```python
from build123d import *

# Parameters (mm, degrees)
SKETCH_1_R      = 2
EXTRUDE_2_DEPTH = 4


with BuildPart() as part:
    # 草图1 → 凸台-拉伸2 (new body)
    with BuildSketch(Plane(origin=(0, 0, 0), x_dir=(1, 0, 0), z_dir=(0, 1, 0))):
        with BuildLine():
            Line((0, -30), (150, -20))
            ThreePointArc((150, -20), (170, 0), (150, 20))
            Line((150, 20), (0, 30))
            ThreePointArc((0, 30), (-30, 0), (0, -30))
        make_face()
        with Locations(Location((0, -17.25, 0), (0, 0, 270))):
            Circle(SKETCH_1_R, mode=Mode.SUBTRACT)
        with Locations(Location((-14.938938215, -8.625, 0), (0, 0, 270))):
            Circle(SKETCH_1_R, mode=Mode.SUBTRACT)
        with Locations(Location((14.938938215, -8.625, 0), (0, 0, 270))):
            Circle(SKETCH_1_R, mode=Mode.SUBTRACT)
        with Locations(Location((-14.938938215, 8.625, 0), (0, 0, 270))):
            Circle(SKETCH_1_R, mode=Mode.SUBTRACT)
        with Locations(Location((14.938938215, 8.625, 0), (0, 0, 270))):
            Circle(SKETCH_1_R, mode=Mode.SUBTRACT)
        with Locations(Location((0, 17.25, 0), (0, 0, 270))):
            Circle(SKETCH_1_R, mode=Mode.SUBTRACT)
        with Locations(Location((141.339745962, -5, 0), (0, 0, 270))):
            Circle(SKETCH_1_R, mode=Mode.SUBTRACT)
        with Locations(Location((150, -10, 0), (0, 0, 270))):
            Circle(SKETCH_1_R, mode=Mode.SUBTRACT)
        with Locations(Location((158.660254038, -5, 0), (0, 0, 270))):
            Circle(SKETCH_1_R, mode=Mode.SUBTRACT)
        with Locations(Location((158.660254038, 5, 0), (0, 0, 270))):
            Circle(SKETCH_1_R, mode=Mode.SUBTRACT)
        with Locations(Location((150, 10, 0), (0, 0, 270))):
            Circle(SKETCH_1_R, mode=Mode.SUBTRACT)
        with Locations(Location((141.339745962, 5, 0), (0, 0, 270))):
            Circle(SKETCH_1_R, mode=Mode.SUBTRACT)
    extrude(amount=EXTRUDE_2_DEPTH)


solid = part.part
```
Read the model definition and answer for the solid it produces. Units are mm, in the model's axes. Coordinates: 2 decimals unless noted, no trailing zeros. Loops run counter-clockwise (first coordinate to the right, second up) from the corner with the lowest first, then second, coordinate; pieces in that order, holes last.
(1) The mould has two halves that part along X. Classify faces 1 (the face through (16.92, 1.97, 8.36)), 2 (the face through (76.05, 1.97, -24.93)), 3 (the face through (69, 4, 0)), 4 (the face through (143.323, 1.972, 4.74)): released by +X, released by -X, zero draft, split by the parting line, or undercut.
Solution:
face 1: undercut
face 2: released by +X
face 3: zero draft
face 4: undercut
(2) The part is cut by section C-C (x = 82). Determine the outline of the cut face in (y, z).
Solution:
outline: (0, -24.53) - (4, -24.53) - (4, 24.53) - (0, 24.53) - close
(3) The part is cut by section A-A (z = 17.25). Determine the outline of the cut face in (x, y), and give its area (3 significant figures).
Solution:
outline: (-24.54, 0) - (-2, 0) - (-2, 4) - (-24.54, 4) - close; (2, 0) - (160.12, 0) - (160.12, 4) - (2, 4) - close
area: 723 mm2
(4) The part is cut by section B-B (y = 0.85). Count the separate pieces of the cut face and the enclosed holes in it, and give its area (3 significant figures).
Solution:
separate pieces: 1
enclosed holes: 12
area: 9,390 mm2
(5) Consider line 1 along Z through (x, y) = (158, 1.45); line 2 along Z through (x, y) = (150, 1.9); line 3 along X through (y, z) = (2.05, -7.5). Determine where each line is inside the solid, lowest interval first.
Solution:
line 1: z = -18.33 to -6.89, -3.11 to 3.11, 6.89 to 18.33
line 2: z = -20 to -12, -8 to 8, 12 to 20
line 3: x = -29.05 to -16.59, -13.29 to 13.29, 16.59 to 168.54
(6) Flat-ended cylindrical pins translate along their axes: pin 1 Ø4.5 at (x, z) = (-14.94, -8.62) entering from -Y; pin 2 Ø1 at (x, y) = (18.5, 3) entering from +Z; pin 3 Ø2 at (x, y) = (15, 2.5) entering from -Z; pin 4 Ø2 at (y, z) = (1.5, 13.5) entering from -X. Find the tip coordinate at first contact, or state that the pin passes through.
Solution:
pin 1: stops at y = 0
pin 2: stops at z = 28.8
pin 3: stops at z = -29.07
pin 4: stops at x = -27.27
